from build123d import *

# Parameters (mm, degrees)
F2_SIZE = 0.25


with BuildPart() as f1:
    # F0 (on Top) → F1 (revolve)
    with BuildSketch(Plane.XY):
        with BuildLine():
            Line((0, 4.484907), (0, 2.205))
            Line((0, 2.205), (2.75, 2.205))
            ThreePointArc((2.75, 2.205), (2.926777, 2.131777), (3, 1.955))
            Line((3, 1.955), (3, 0.85))
            ThreePointArc((3, 0.85), (3.029289, 0.779289), (3.1, 0.75))
            Line((3.1, 0.75), (4.46, 0.75))
            ThreePointArc((4.46, 0.75), (4.530711, 0.779289), (4.56, 0.85))
            Line((4.56, 0.85), (4.56, 3.5339))
            ThreePointArc((4.56, 3.5339), (4.852893, 4.241007), (5.56, 4.5339))
            Line((5.56, 4.5339), (32.766, 4.5339))
            Line((32.766, 4.5339), (32.766, 4.8133))
            Line((32.766, 4.8133), (3.13, 4.8133))
            Line((3.13, 4.8133), (1.9, 4.215))
            Line((1.9, 4.215), (1.14, 4.215))
            Line((1.14, 4.215), (1.14, 4.8))
            Line((1.14, 4.8), (0.45, 4.8))
            Line((0.45, 4.8), (0, 4.484907))
        make_face()
    revolve(axis=Axis((16.383, 0, 0), (-1, 0, 0)))

    # F2
    f2_edges = [f1.edges().sort_by_distance(p)[0] for p in [
        (0, -2.205, 0),
    ]]
    chamfer(f2_edges, length=F2_SIZE)


solid = f1.part
Work out the finished part from the listing and answer in its coordinate system (mm). A direction names the side the tool comes from. Give positions to 0.01 mm unless a question says otherwise; leave off trailing zeros. Order: outer loops, then holes, each group sorted by start corner. A loop starts at its lowest first (then second) coordinate and runs counter-clockwise, first axis right, second up. Notation, with made-up numbers: (82.25, -21.75) -> (139.25, -21.75) arc R27 ccw to (139.25, 15.25) -> close; hole circle Ø11 at (48, 43). An arc over 180 degrees is marked (long way). Answer as a JSON object with one key per item and string values. Group by question number.
1. Consider line 1 along Z through (x, y) = (3.4, 0); line 2 along Y through (x, z) = (1, 0) (3 decimals). Determine where each line is inside the solid, lowest interval first. Write a range as [from, to].
2. Flat-ended cylindrical pins translate along their axes: pin 1 Ø5 at (y, z) = (-1.5, 1) entering from +X; pin 2 Ø2 at (y, z) = (-0.5, 0.5) entering from -X; pin 3 Ø2 at (y, z) = (-0.5, 0) entering from +X. Find the tip coordinate at first contact, or state that the pin passes through.
3. Section A-A on x = 31.5 is taken. Determine the outline of the cut face in (y, z), plus the area to 3 significant figures.
4. A tool of negligible diameter and unlimited length cuts with its end or side. For faces 1 (the cylindrical face through (17.74, -3.82, 2.93)), 2 (the flat face through (1.14, -2, 4)), 3 (the cylindrical face through (19.353, 4.325, -1.362)), 4 (the flat face through (3, 0, 1)), from which of +Z, -Z, +X, -X, +Y, -Y can it reach the whole face along a straight path? Write none if from no direction.
5. The mould has two halves that part along X. Classify faces 5 (the cylindrical face through (1.515, -0.914, 4.115)), 6 (the cylindrical face through (1.518, 2.103, -0.662)), 7 (the flat face through (0, 2, 2)): released by +X, released by -X, zero draft, split by the parting line, or undercut.
Result sheet:
{
 "1": {"line 1": "z = [-4.81, -0.75], [0.75, 4.81]", "line 2": "y = [-4.8, -2.205], [2.205, 4.8]"},
 "2": {"pin 1": "stops at x = 4.92", "pin 2": "stops at x = 3", "pin 3": "stops at x = 4.56"},
 "3": {"outline": "circle Ø9.63 at (0, 0); hole circle Ø9.07 at (0, 0)", "area": "8.20 mm^2"},
 "4": {"face 1": "+X, -X", "face 2": "none", "face 3": "+X", "face 4": "-X"},
 "5": {"face 5": "undercut", "face 6": "zero draft", "face 7": "released by -X"}
}
